Verification items for the finished model (mm, model axes). A direction names the side the tool comes from. Round coordinates to 2 decimals unless told otherwise and drop trailing zeros. Order: outer loops, then holes, each group sorted by start corner. A loop starts at its lowest first (then second) coordinate and runs counter-clockwise, first axis right, second up. Notation, with made-up numbers: (88, 19.25) -> (118, 19.25) arc R14 cw to (118, 45.25) -> close; hole circle Ø6 at (85, 36.25). An arc over 180 degrees is marked (long way). Put each result on its own line as item: value.
from build123d import *

# Parameters (mm, degrees)
SKETCH_1_R            = 10
EXTRUDE_1_DEPTH       = 2
SKETCH_2_R            = 4.5
EXTRUDE_2_DEPTH       = 2.5
SKETCH_3_R            = 2.95
CUT_EXTRUDE_1_DEPTH   = 4
HOLE_WIZARD_3_0_3_1_D = 3


with BuildPart() as part:
    # 草图1 → 凸台-拉伸1 (new body)
    with BuildSketch(Plane(origin=(0, 0, 0), x_dir=(1, 0, 0), z_dir=(0, 1, 0))):
        with Locations(Location((0, 0, 0), (0, 0, 270))):
            Circle(SKETCH_1_R)
    extrude(amount=EXTRUDE_1_DEPTH)

    # 草图2 → 凸台-拉伸2 (add)
    with BuildSketch(Plane(origin=(0, 2, 0), x_dir=(1, 0, 0), z_dir=(0, 1, 0))):
        with Locations(Location((0, 0, 0), (0, 0, 270))):
            Circle(SKETCH_2_R)
    extrude(amount=EXTRUDE_2_DEPTH)

    # 草图3 → 切除-拉伸1 (cut)
    with BuildSketch(Plane(origin=(0, 4.5, 0), x_dir=(1, 0, 0), z_dir=(0, 1, 0))):
        with Locations(Location((0, 0, 0), (0, 0, 270))):
            Circle(SKETCH_3_R)
    extrude(amount=-CUT_EXTRUDE_1_DEPTH, mode=Mode.SUBTRACT)

    # Ø3.0 (3) 直径孔1 (through all)
    with Locations(Plane(origin=(0, 2, 0), x_dir=(1, 0, 0), z_dir=(0, 1, 0))):
        with Locations((0, 7), (7, 0), (0, -7), (-7, 0), (0, 0)):
            Hole(HOLE_WIZARD_3_0_3_1_D / 2)


solid = part.part
Item 1: Section check D-D on y = 3.3. Record the boundary of the cut face in (x, z), then the cut area to 3 significant figures.
Check sheet entries:
outline: circle Ø9 at (0, 0); hole circle Ø5.9 at (0, 0)
area: 36.3 mm^2
Item 2: Material ranges on L1, parallel to X at y = 3.15, z = 0; L2, parallel to Y at x = -1, z = 1.75; L3, parallel to Y at x = 0.5, z = 8.75, recorded low to high. Write a range as [from, to].
Check sheet entries:
L1: x = [-4.5, -2.95], [2.95, 4.5]
L2: y = [0, 0.5]
L3: y = [0, 2]
Item 3: Section check C-C on z = -5.75. Record the boundary of the cut face in (x, y), then the cut area to 3 significant figures.
Check sheet entries:
outline: (-8.18, 0) -> (-0.83, 0) -> (-0.83, 2) -> (-8.18, 2) -> close; (0.83, 0) -> (8.18, 0) -> (8.18, 2) -> (0.83, 2) -> close
area: 29.4 mm^2
Item 4: Tool access check on faces 4 (the cylindrical face through (0.325, 0.986, -5.536)), 5 (the flat face through (-1.3, 0.5, 1.3)). Record the directions out of +Z, -Z, +X, -X, +Y, -Y that give a thin tool (end or side, any length) a straight path to the whole face; none if there is none.
Check sheet entries:
face 4: +Y, -Y
face 5: +Y
Item 5: Section check B-B on z = -1. Record the boundary of the cut face in (x, y), then the cut area to 3 significant figures.
Check sheet entries:
outline: (-9.95, 0) -> (-8.12, 0) -> (-8.12, 2) -> (-9.95, 2) -> close; (-5.88, 0) -> (-1.12, 0) -> (-1.12, 0.5) -> (-2.78, 0.5) -> (-2.78, 4.5) -> (-4.39, 4.5) -> (-4.39, 2) -> (-5.88, 2) -> close; (1.12, 0) -> (5.88, 0) -> (5.88, 2) -> (4.39, 2) -> (4.39, 4.5) -> (2.78, 4.5) -> (2.78, 0.5) -> (1.12, 0.5) -> close; (8.12, 0) -> (9.95, 0) -> (9.95, 2) -> (8.12, 2) -> close
area: 29.5 mm^2
Item 6: Release check for a two-part mould opening along X. For faces 1 (the flat face through (-3, 4.5, 1)), 2 (the cylindrical face through (-2.88, 2.53, -0.64)), 3 (the cylindrical face through (1.352, 3.232, 4.292)) record: +X half, -X half, draft (parallel to the pull), parting line (faces both ways), or undercut.
Check sheet entries:
face 1: draft
face 2: undercut
face 3: parting line
Item 7: Gauge pin test, flat ends, axial feed: pin 1 Ø1.5 at (x, z) = (-6.5, 1.5) entering from +Y; pin 2 Ø1 at (x, y) = (-4, 2) entering from -Z; pin 3 Ø1.8 at (x, z) = (0, -7) entering from +Y (1 decimal). Record the tip position at first contact, or that the pin passes through.
Check sheet entries:
pin 1: stops at y = 2
pin 2: stops at z = -9.37
pin 3: passes through
Item 8: Section check A-A on x = 6.75. Record the boundary of the cut face in (y, z), then the cut area to 3 significant figures.
Check sheet entries:
outline: (0, -7.38) -> (2, -7.38) -> (2, -1.48) -> (0, -1.48) -> close; (0, 1.48) -> (2, 1.48) -> (2, 7.38) -> (0, 7.38) -> close
area: 23.6 mm^2
